Check sheet for the modelled part. Datum: model origin and axes. Units: mm. Round coordinates to 2 decimals unless told otherwise and drop trailing zeros. Order: outer loops, then holes, each group sorted by start corner. A loop starts at its lowest first (then second) coordinate and runs counter-clockwise, first axis right, second up.
from build123d import *

# Parameters (mm, degrees)
ESQUISSE1_W             = 1974
ESQUISSE1_H             = 1700
ESQUISSE1_W_2           = 930
ESQUISSE1_H_2           = 1624
BOSS_EXTRU_1_DEPTH      = 63
ESQUISSE2_R             = 8
ENL_V_MAT_EXTRU_1_DEPTH = 2606.886605361


with BuildPart() as part:
    # Esquisse1 → Boss.-Extru.1 (new body)
    with BuildSketch(Plane.XY):
        with Locations((987, 850)):
            Rectangle(ESQUISSE1_W, ESQUISSE1_H)
        with Locations((1471, 850)):
            Rectangle(ESQUISSE1_W_2, ESQUISSE1_H_2, mode=Mode.SUBTRACT)
        with Locations((503, 850)):
            Rectangle(ESQUISSE1_W_2, ESQUISSE1_H_2, mode=Mode.SUBTRACT)
    extrude(amount=BOSS_EXTRU_1_DEPTH)

    # Esquisse2 → Enlèv. mat.-Extru.1 (cut, through all)
    with BuildSketch(Plane(origin=(1974, 0, 0), x_dir=(0, 0, -1), z_dir=(1, 0, 0))):
        with Locations((-31.5, 850)):
            Circle(ESQUISSE2_R)
    extrude(amount=-ENL_V_MAT_EXTRU_1_DEPTH, mode=Mode.SUBTRACT)


solid = part.part
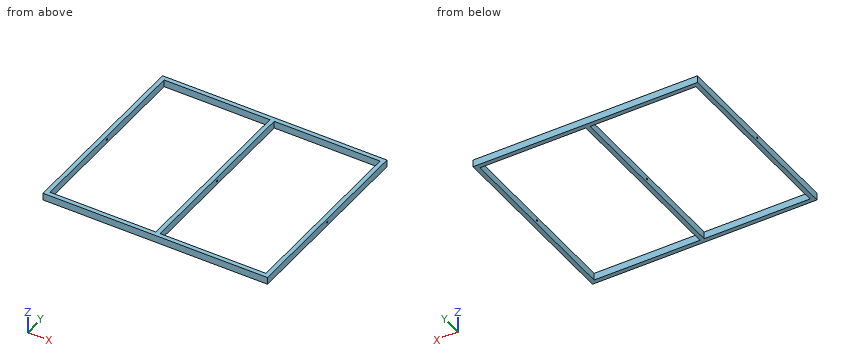
1) Sectioned sample at B-B on y = 1078.5. Record the cut outline in (x, z), and give its area (3 significant figures).
2) Scan lines: line 1 (X direction, y = 991.5, z = 48); line 2 (Y direction, x = 27, z = 31.5); line 3 (Y direction, x = 388, z = 36.5). Record each from-to range of solid material in increasing order.
3) Sectioned sample at C-C on z = 13.5. Record the cut outline in (x, y).
4) Sectioned sample at A-A on x = 1063. Record the cut outline in (y, z).
5) Gauge pin test, flat end, axial feed: pin 1 (1 mm diameter, centred on x = 337.5, z = 15, fed in from -Y). Record the tip position at first contact, or that the pin passes through.
Values found:
1. outline: (0, 0) - (38, 0) - (38, 63) - (0, 63) - close; (968, 0) - (1006, 0) - (1006, 63) - (968, 63) - close; (1936, 0) - (1974, 0) - (1974, 63) - (1936, 63) - close
1. area: 7,180 mm2
2. line 1: x = 0 to 38, 968 to 1006, 1936 to 1974
2. line 2: y = 0 to 842, 858 to 1700
2. line 3: y = 0 to 38, 1662 to 1700
3. outline: (0, 0) - (1974, 0) - (1974, 1700) - (0, 1700) - close; hole (38, 38) - (968, 38) - (968, 1662) - (38, 1662) - close; hole (1006, 38) - (1936, 38) - (1936, 1662) - (1006, 1662) - close
4. outline: (0, 0) - (38, 0) - (38, 63) - (0, 63) - close; (1662, 0) - (1700, 0) - (1700, 63) - (1662, 63) - close
5. pin 1: stops at y = 0
